The model under review builds one solid part; all positions refer to its coordinate system, in mm. A direction names the side the tool comes from. Coordinates: 2 decimals unless noted, no trailing zeros. Order: outer loops, then holes, each group sorted by start corner. A loop starts at its lowest first (then second) coordinate and runs counter-clockwise, first axis right, second up.
```python
from build123d import *

# Parameters (mm, degrees)
F0_W      = 124.8
F0_H      = 81
F1_DEPTH  = 25
F2_W      = 122.5
F2_H      = 78.7
F3_DEPTH  = 3
F4_W      = 120.8
F4_H      = 77
F5_DEPTH  = 26
F6_W      = 10
F6_H      = 10
F7_DEPTH  = 24.4
F8_R      = 1.5
F9_DEPTH  = 4.8
F10_W     = 26
F10_H     = 45
F10_W_2   = 17
F10_H_2   = 12.8
F10_W_3   = 12.8
F10_H_3   = 30.7
F11_DEPTH = 2.001
F12_R     = 3
F13_DEPTH = 4
F14_R     = 1.5
F15_DEPTH = 4.8
F16_W     = 12
F16_H     = 57
F17_DEPTH = 6
F18_R     = 1.5
F19_DEPTH = 4.8
F20_W     = 26
F20_H     = 16
F21_DEPTH = 6
F22_R     = 1.5
F23_DEPTH = 4.8


with BuildPart() as f1:
    # F0 (on Top) → F1 (new body)
    with BuildSketch(Plane.XY):
        Rectangle(F0_W, F0_H)
    extrude(amount=F1_DEPTH)

    # F2 (on face) → F3 (join)
    with BuildSketch(Plane.XY.offset(25)):
        Rectangle(F2_W, F2_H)
    extrude(amount=F3_DEPTH)

    # F4 (on face) → F5 (cut)
    with BuildSketch(Plane.XY.offset(28)):
        Rectangle(F4_W, F4_H)
    extrude(amount=-F5_DEPTH, mode=Mode.SUBTRACT)

    # F6 (on face) → F7 (join)
    with BuildSketch(Plane.XY.offset(2)):
        with Locations((-55.4, 33.5)):
            Rectangle(F6_W, F6_H)
        with Locations((-55.4, -33.5)):
            Rectangle(F6_W, F6_H)
        with Locations((55.4, -33.5)):
            Rectangle(F6_W, F6_H)
        with Locations((55.4, 33.5)):
            Rectangle(F6_W, F6_H)
    extrude(amount=F7_DEPTH)

    # F8 (on face) → F9 (cut)
    with BuildSketch(Plane.XY.offset(26.4)):
        with Locations((-55, 33.5)):
            Circle(F8_R)
        with Locations((-55, -33.5)):
            Circle(F8_R)
        with Locations((55, -33.5)):
            Circle(F8_R)
        with Locations((55, 33.5)):
            Circle(F8_R)
    extrude(amount=-F9_DEPTH, mode=Mode.SUBTRACT)

    # F10 (on face) → F11 (cut, through all)
    with BuildSketch(Plane.XY.offset(2)):
        with Locations((44.4, 5)):
            Rectangle(F10_W, F10_H)
        with Locations((24.9, -29.1)):
            Rectangle(F10_W_2, F10_H_2)
        with Locations((9.5, 0)):
            Rectangle(F10_W_3, F10_H_3)
    extrude(amount=-F11_DEPTH, mode=Mode.SUBTRACT)

    # F12 (on face) → F13 (join)
    with BuildSketch(Plane.XY.offset(2)):
        with Locations((24.4, 13.2)):
            Circle(F12_R)
        with Locations((-34.6, 13.2)):
            Circle(F12_R)
        with Locations((-34.6, -15.8)):
            Circle(F12_R)
        with Locations((24.4, -15.8)):
            Circle(F12_R)
        with Locations((-43.4, 31.5)):
            Circle(F12_R)
        with Locations((-43.4, 22.5)):
            Circle(F12_R)
        with Locations((-20.4, 31.5)):
            Circle(F12_R)
        with Locations((-5.4, 31.5)):
            Circle(F12_R)
        with Locations((11.6, 31.5)):
            Circle(F12_R)
    extrude(amount=F13_DEPTH)

    # F14 (on face) → F15 (cut)
    with BuildSketch(Plane.XY.offset(2)):
        with Locations((-34.6, -15.8)):
            Circle(F14_R)
        with Locations((24.4, -15.8)):
            Circle(F14_R)
        with Locations((-34.6, 13.2)):
            Circle(F14_R)
        with Locations((24.4, 13.2)):
            Circle(F14_R)
        with Locations((11.6, 31.5)):
            Circle(F14_R)
        with Locations((-5.4, 31.5)):
            Circle(F14_R)
        with Locations((-20.4, 31.5)):
            Circle(F14_R)
        with Locations((-43.4, 22.5)):
            Circle(F14_R)
        with Locations((-43.4, 31.5)):
            Circle(F14_R)
    extrude(amount=F15_DEPTH, mode=Mode.SUBTRACT)

    # F16 (on face) → F17 (join)
    with BuildSketch(Plane.XY.offset(2)):
        with Locations((-54.4, 0)):
            Rectangle(F16_W, F16_H)
    extrude(amount=F17_DEPTH)

    # F18 (on face) → F19 (cut)
    with BuildSketch(Plane.XY.offset(8)):
        with Locations((-54.4, 0)):
            Circle(F18_R)
    extrude(amount=-F19_DEPTH, mode=Mode.SUBTRACT)

    # F20 (on face) → F21 (join)
    with BuildSketch(Plane.XY.offset(2)):
        with Locations((-22.927424, -30.5)):
            Rectangle(F20_W, F20_H)
    extrude(amount=F21_DEPTH)

    # F22 (on face) → F23 (cut)
    with BuildSketch(Plane.XY.offset(8)):
        with Locations((-22.927424, -25)):
            Circle(F22_R)
        with Locations((-22.927424, -36)):
            Circle(F22_R)
    extrude(amount=-F23_DEPTH, mode=Mode.SUBTRACT)


solid = f1.part
```
(1) For pin 1 Ø6.5 at (x, y) = (23, 12.5) entering from +Z; pin 2 Ø0.9 at (x, y) = (-54.5, -33.5) entering from +Z; pin 3 Ø6 at (x, y) = (0, -2.5) entering from +Z, all flat-tipped, find the tip position at first contact; note any pin that passes through.
A:
pin 1: stops at z = 6
pin 2: stops at z = 21.6
pin 3: stops at z = 2
(2) We need section C-C, the plane x = 11.6. Write out the cut boundary in (y, z).
A:
outline: (-40.5, 0) - (-15.35, 0) - (-15.35, 2) - (-38.5, 2) - (-38.5, 28) - (-39.35, 28) - (-39.35, 25) - (-40.5, 25) - close; (15.35, 0) - (40.5, 0) - (40.5, 25) - (39.35, 25) - (39.35, 28) - (38.5, 28) - (38.5, 2) - (34.5, 2) - (34.5, 6) - (33, 6) - (33, 2) - (30, 2) - (30, 6) - (28.5, 6) - (28.5, 2) - (15.35, 2) - close
(3) We need section B-B, the plane y = 7. Write out the cut boundary in (x, z).
A:
outline: (-62.4, 0) - (3.1, 0) - (3.1, 2) - (-48.4, 2) - (-48.4, 8) - (-60.4, 8) - (-60.4, 28) - (-61.25, 28) - (-61.25, 25) - (-62.4, 25) - close; (15.9, 0) - (31.4, 0) - (31.4, 2) - (15.9, 2) - close; (57.4, 0) - (62.4, 0) - (62.4, 25) - (61.25, 25) - (61.25, 28) - (60.4, 28) - (60.4, 2) - (57.4, 2) - close
(4) Draft analysis for pull direction Y (two halves, no side actions). For faces 1 (the face through (-57, -33, 26.4)), 2 (the face through (-1, -39.35, 26)), 3 (the face through (-1, 39.35, 26)), state which applies: released by +Y, released by -Y, zero draft, split by the parting line, or undercut.
A:
face 1: undercut
face 2: released by -Y
face 3: released by +Y
(5) We need section A-A, the plane z = 23.75. Write out the cut boundary in (x, y), and give its area (3 significant figures).
A:
outline: (-62.4, -40.5) - (62.4, -40.5) - (62.4, 40.5) - (-62.4, 40.5) - close; hole (-60.4, -28.5) - (-50.4, -28.5) - (-50.4, -38.5) - (50.4, -38.5) - (50.4, -28.5) - (60.4, -28.5) - (60.4, 28.5) - (50.4, 28.5) - (50.4, 38.5) - (-50.4, 38.5) - (-50.4, 28.5) - (-60.4, 28.5) - close; hole circle Ø3 at (-55, -33.5); hole circle Ø3 at (-55, 33.5); hole circle Ø3 at (55, -33.5); hole circle Ø3 at (55, 33.5)
area: 1,180 mm2
(6) Wall thickness on probe 1 along Y at (x, z) = (24.4, 3.25); probe 2 along X at (y, z) = (-31, 20.25); probe 3 along Y at (x, z) = (-21.5, 17.25): over which ranges is each line inside the solid? List them lowest first.
A:
probe 1: y = -40.5 to -38.5, -18.8 to -17.3, -14.3 to -12.8, 10.2 to 11.7, 14.7 to 16.2, 38.5 to 40.5
probe 2: x = -62.4 to -50.4, 50.4 to 62.4
probe 3: y = -40.5 to -38.5, 38.5 to 40.5
(7) We need section D-D, the plane y = -25. Write out the cut boundary in (x, z).
A:
outline: (-62.4, 0) - (16.4, 0) - (16.4, 2) - (-9.93, 2) - (-9.93, 8) - (-21.43, 8) - (-21.43, 3.2) - (-24.43, 3.2) - (-24.43, 8) - (-35.93, 8) - (-35.93, 2) - (-48.4, 2) - (-48.4, 8) - (-60.4, 8) - (-60.4, 28) - (-61.25, 28) - (-61.25, 25) - (-62.4, 25) - close; (33.4, 0) - (62.4, 0) - (62.4, 25) - (61.25, 25) - (61.25, 28) - (60.4, 28) - (60.4, 2) - (33.4, 2) - close
(8) Machinability: for faces 4 (the face through (-54.31, -34.83, 24.03)), 5 (the face through (-15, 1, 0)), which of the approach directions +Z, -Z, +X, -X, +Y, -Y give a long, thin tool a straight path to every point of the face, cutting with its end or side? Answer none if there is none.
A:
face 4: +Z
face 5: -Z, +X, -X, +Y, -Y
